```python
from build123d import *

# Parameters (mm, degrees)
SKETCH1_W           = 163
SKETCH1_H           = 50
BOSS_EXTRUDE1_DEPTH = 5
SKETCH6_W           = 163
SKETCH6_H           = 5
BOSS_EXTRUDE2_DEPTH = 129
CUT_EXTRUDE1_DEPTH  = 164.166326183
FILLET1_R           = 5
FILLET2_R           = 20
CUT_EXTRUDE2_DEPTH  = 155.622928594
CUT_EXTRUDE3_DEPTH  = 155.622928594


with BuildPart() as part:
    # Sketch1 → Boss-Extrude1 (new body)
    with BuildSketch(Plane(origin=(0, 0, 0), x_dir=(1, 0, 0), z_dir=(0, 1, 0))):
        Rectangle(SKETCH1_W, SKETCH1_H)
    extrude(amount=BOSS_EXTRUDE1_DEPTH)

    # Sketch6 → Boss-Extrude2 (add)
    with BuildSketch(Plane(origin=(0, 5, 0), x_dir=(1, 0, 0), z_dir=(0, 1, 0))):
        with Locations((0, 22.5)):
            Rectangle(SKETCH6_W, SKETCH6_H)
    extrude(amount=BOSS_EXTRUDE2_DEPTH)

    # Sketch7 → Cut-Extrude1 (cut, through all)
    with BuildSketch(Plane.XY.offset(-20)):
        with BuildLine():
            ThreePointArc((-32.33968901, 59.421555555), (70.67427925, 69.5), (-32.33968901, 79.578444445))
            ThreePointArc((-32.33968901, 79.578444445), (-43.452284877, 69.5), (-32.33968901, 59.421555555))
        make_face()
    extrude(amount=-CUT_EXTRUDE1_DEPTH, mode=Mode.SUBTRACT)

    # Fillet1
    fillet1_edges = [part.edges().sort_by_distance(p)[0] for p in [
        (-32.33968901, 59.421555555, -22.5),
        (-32.33968901, 79.578444445, -22.5),
    ]]
    fillet(fillet1_edges, radius=FILLET1_R)

    # Fillet2
    fillet2_edges = [part.edges().sort_by_distance(p)[0] for p in [
        (-81.5, 134, -22.5),
        (81.5, 134, -22.5),
    ]]
    fillet(fillet2_edges, radius=FILLET2_R)

    # Sketch9 → Cut-Extrude2 (cut, through all)
    with BuildSketch(Plane(origin=(0, 5, 0), x_dir=(1, 0, 0), z_dir=(0, 1, 0))):
        with BuildLine():
            Line((-61, 10), (-61, -20))
            ThreePointArc((-61, -20), (-64.5, -23.5), (-68, -20))
            Line((-68, -20), (-68, 10))
            ThreePointArc((-68, 10), (-64.5, 13.5), (-61, 10))
        make_face()
    cut_extrude2 = extrude(amount=-CUT_EXTRUDE2_DEPTH, mode=Mode.SUBTRACT)

    # Mirror3: Cut-Extrude2 across plane
    add(cut_extrude2.mirror(Plane(origin=(0, 0, 0), x_dir=(0, 0, 1), z_dir=(1, 0, 0))), mode=Mode.SUBTRACT)

    # Sketch10 → Cut-Extrude3 (cut, through all)
    with BuildSketch(Plane(origin=(0, 5, 0), x_dir=(1, 0, 0), z_dir=(0, 1, 0))):
        with BuildLine():
            Line((3.5, 10), (3.5, -20))
            ThreePointArc((3.5, -20), (0, -23.5), (-3.5, -20))
            Line((-3.5, -20), (-3.5, 10))
            ThreePointArc((-3.5, 10), (0, 13.5), (3.5, 10))
        make_face()
    extrude(amount=-CUT_EXTRUDE3_DEPTH, mode=Mode.SUBTRACT)


solid = part.part
```
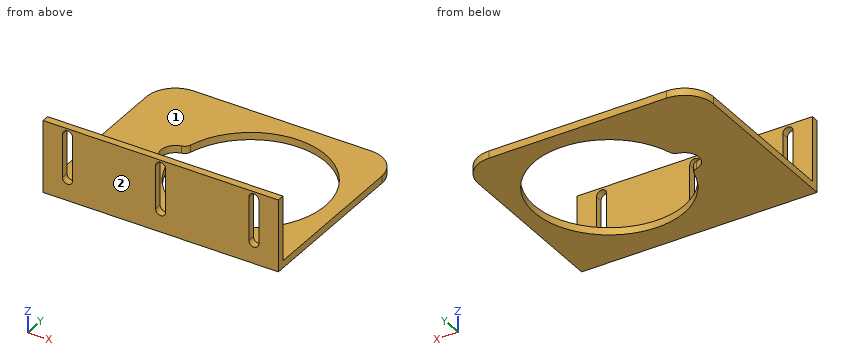
The listing builds one solid part. Answer for the finished solid, in the listing's coordinates (mm). Face numbers are marked on the shaded views. A direction names the side the tool comes from. Give positions to 0.01 mm unless a question says otherwise; leave off trailing zeros. Write each loop counter-clockwise with the first axis right and the second up, starting at its lowest first coordinate (ties: lowest second). Pieces come first, ordered by that corner, then holes. Notation, with made-up numbers: (-1.5, 54.5) - (53.5, 54.5) arc R33 ccw to (53.5, 85.5) - close; hole circle Ø3 at (65.5, 12). An arc over 180 degrees is marked (long way). Use one line per item in the form item = value. Start each with the question number.
1) Find section A-A on z = 4.5. Determine the outline of the cut face in (x, y).
2) Flat-ended cylindrical pins translate along their axes: pin 1 Ø3 at (x, y) = (-55.5, 41) entering from +Z; pin 2 Ø3 at (x, z) = (31, 10.5) entering from +Y. Find the tip coordinate at first contact, or state that the pin passes through.
3) Find section C-C on y = 47. Determine the outline of the cut face in (x, z), plus the area to 3 significant figures.
4) Find section D-D on x = 65.5. Determine the outline of the cut face in (y, z).
5) Find section B-B on x = -64.5. Determine the outline of the cut face in (y, z), plus the area to 3 significant figures.
6) Consider line 1 along X through (y, z) = (69, -23); line 2 along Y through (x, z) = (58, -14); line 3 along Z through (x, y) = (-38.5, 18.5). Determine where each line is inside the solid, lowest interval first. Write a range as from..to.
7) A tool of negligible diameter and unlimited length cuts with its end or side. For the marked faces 1 and 2, from which of +Z, -Z, +X, -X, +Y, -Y can it reach the whole face along a straight path? Write none if from no direction.
Geometry results:
q1.outline = (-81.5, 0) - (-68, 0) - (-68, 5) - (-81.5, 5) - close; (-61, 0) - (-3.5, 0) - (-3.5, 5) - (-61, 5) - close; (3.5, 0) - (61, 0) - (61, 5) - (3.5, 5) - close; (68, 0) - (81.5, 0) - (81.5, 5) - (68, 5) - close
q2.pin_1 = -20
q2.pin_2 = 5
q3.outline = (-81.5, -25) - (-28.21, -25) - (-28.21, -20) - (-81.5, -20) - close; (65.55, -25) - (81.5, -25) - (81.5, -20) - (65.55, -20) - close
q3.area = 346 mm2
q4.outline = (0, -25) - (46.89, -25) - (46.89, -20) - (5, -20) - (5, -13.35) - (0, -13.35) - close; (0, 23.35) - (5, 23.35) - (5, 25) - (0, 25) - close; (92.11, -25) - (133.6, -25) - (133.6, -20) - (92.11, -20) - close
q5.outline = (0, -25) - (133.77, -25) - (133.77, -20) - (5, -20) - (5, -13.5) - (0, -13.5) - close; (0, 23.5) - (5, 23.5) - (5, 25) - (0, 25) - close
q5.area = 709 mm2
q6.line_1 = -81.5..-43.44, 70.67..81.5
q6.line_2 = 0..5
q6.line_3 = -25..-20
q7.face_1 = +Z, +X, -X, +Y
q7.face_2 = +Z, -Z, +X, -X, -Y
